from build123d import *

# Parameters (mm, degrees)
ESQUISSE1_W                  = 40
ESQUISSE1_H                  = 10
BOSS_EXTRU_1_DEPTH           = 20
ESQUISSE2_R                  = 1.75
ENL_V_MAT_EXTRU_1_DEPTH      = 1
ENL_V_MAT_EXTRU_1_DEPTH_BACK = 21
ESQUISSE3_R                  = 3.15
ENL_V_MAT_EXTRU_2_DEPTH      = 1
ENL_V_MAT_EXTRU_2_DEPTH_BACK = 11
ESQUISSE4_R                  = 3.65
ENL_V_MAT_EXTRU_3_DEPTH      = 1
CONG_1_R                     = 5


with BuildPart() as part:
    # Esquisse1 → Boss.-Extru.1 (new body)
    with BuildSketch(Plane.XY):
        with Locations((20, 5)):
            Rectangle(ESQUISSE1_W, ESQUISSE1_H)
    extrude(amount=BOSS_EXTRU_1_DEPTH)

    # Esquisse2 → Enlèv. mat.-Extru.1 (cut, two sides)
    with BuildSketch(Plane.XY.offset(20)) as enl_v_mat_extru_1_sk:
        with Locations((20, 5)):
            Circle(ESQUISSE2_R)
        with Locations((11, 5)):
            Circle(ESQUISSE2_R)
        with Locations((29, 5)):
            Circle(ESQUISSE2_R)
    extrude(amount=ENL_V_MAT_EXTRU_1_DEPTH, mode=Mode.SUBTRACT)
    extrude(enl_v_mat_extru_1_sk.sketch, amount=-ENL_V_MAT_EXTRU_1_DEPTH_BACK, mode=Mode.SUBTRACT)

    # Esquisse3 → Enlèv. mat.-Extru.2 (cut, two sides)
    with BuildSketch(Plane(origin=(0, 10, 0), x_dir=(1, 0, 0), z_dir=(0, 1, 0))) as enl_v_mat_extru_2_sk:
        with Locations((5, -10)):
            Circle(ESQUISSE3_R)
        with Locations((35, -10)):
            Circle(ESQUISSE3_R)
    extrude(amount=ENL_V_MAT_EXTRU_2_DEPTH, mode=Mode.SUBTRACT)
    extrude(enl_v_mat_extru_2_sk.sketch, amount=-ENL_V_MAT_EXTRU_2_DEPTH_BACK, mode=Mode.SUBTRACT)

    # Esquisse4 → Enlèv. mat.-Extru.3 (cut)
    with BuildSketch(Plane(origin=(0, 10, 0), x_dir=(1, 0, 0), z_dir=(0, 1, 0))):
        with Locations((5, -10)):
            Circle(ESQUISSE4_R)
        with Locations((35, -10)):
            Circle(ESQUISSE4_R)
    extrude(amount=-ENL_V_MAT_EXTRU_3_DEPTH, mode=Mode.SUBTRACT)

    # Congé1
    cong_1_edges = [part.edges().sort_by_distance(p)[0] for p in [
        (40, 5, 20),
        (0, 5, 20),
        (40, 5, 0),
        (0, 5, 0),
    ]]
    fillet(cong_1_edges, radius=CONG_1_R)


solid = part.part
Work out the finished part from the listing and answer in its coordinate system (mm). A direction names the side the tool comes from. Give positions to 0.01 mm unless a question says otherwise; leave off trailing zeros. Order: outer loops, then holes, each group sorted by start corner. A loop starts at its lowest first (then second) coordinate and runs counter-clockwise, first axis right, second up. Notation, with made-up numbers: (-18, -14.75) -> (10, -14.75) arc R27 ccw to (10, 22.25) -> close; hole circle Ø8 at (-13, 82). An arc over 180 degrees is marked (long way). One line per item, written item: value.
Item 1: Straight lines are drawn through the part: probe 1 along X at (y, z) = (9.5, 10); probe 2 along X at (y, z) = (5.75, 17.5); probe 3 along X at (y, z) = (2.5, 10). For each, find the intervals that lie inside material, in ascending order.
Answer sheet:
probe 1: 0 to 1.35, 8.65 to 31.35, 38.65 to 40
probe 2: 0.67 to 9.42, 12.58 to 18.42, 21.58 to 27.42, 30.58 to 39.33
probe 3: 0 to 1.85, 8.15 to 31.85, 38.15 to 40
Item 2: Find section C-C, the plane x = 11. Give the vertices of the cut face in (y, z), plus the area to 3 significant figures.
Answer sheet:
outline: (0, 0) -> (3.25, 0) -> (3.25, 20) -> (0, 20) -> close; (6.75, 0) -> (10, 0) -> (10, 20) -> (6.75, 20) -> close
area: 130 mm²
Item 3: Find section D-D, the plane y = 7.25. Give the vertices of the cut face in (x, z), plus the area to 3 significant figures.
Answer sheet:
outline: (0, 5) arc R5 ccw to (5, 0) -> (35, 0) arc R5 ccw to (40, 5) -> (40, 15) arc R5 ccw to (35, 20) -> (5, 20) arc R5 ccw to (0, 15) -> close; hole circle Ø6.3 at (5, 10); hole circle Ø6.3 at (35, 10)
area: 716 mm²
Item 4: Find section A-A, the plane z = 10. Give the vertices of the cut face in (x, y), plus the area to 3 significant figures.
Answer sheet:
outline: (0, 0) -> (1.85, 0) -> (1.85, 9) -> (1.35, 9) -> (1.35, 10) -> (0, 10) -> close; (8.15, 0) -> (31.85, 0) -> (31.85, 9) -> (31.35, 9) -> (31.35, 10) -> (8.65, 10) -> (8.65, 9) -> (8.15, 9) -> close; (38.15, 0) -> (40, 0) -> (40, 10) -> (38.65, 10) -> (38.65, 9) -> (38.15, 9) -> close; hole circle Ø3.5 at (11, 5); hole circle Ø3.5 at (20, 5); hole circle Ø3.5 at (29, 5)
area: 243 mm²
Item 5: A flat-ended cylindrical pin translates along its axis: P1, Ø2, axis at x = 33.5, z = 8, coming from the +Y side. Find the tip coordinate at first contact, or state that the pin passes through.
Answer sheet:
P1: y = 9
Item 6: Determine the mould class of faces 3 (the cylindrical face through (11.81, 3.45, 10.14)), 4 (the cylindrical face through (38, 5, 1)), 5 (the cylindrical face through (1, 5, 2)) for opening direction X: released by +X, released by -X, zero draft, split by the parting line, or undercut.
Answer sheet:
face 3: undercut
face 4: released by +X
face 5: released by -X
Item 7: A tool of negligible diameter and unlimited length cuts with its end or side. For faces 1 (the cylindrical face through (6.68, 9.51, 13.24)), 2 (the cylindrical face through (4.59, 4.563, 6.877)), from which of +Z, -Z, +X, -X, +Y, -Y can it reach the whole face along a straight path? Write none if from no direction.
Answer sheet:
face 1: +Y
face 2: +Y, -Y
Item 8: Find section B-B, the plane y = 5. Give the vertices of the cut face in (x, z).
Answer sheet:
outline: (0, 5) arc R5 ccw to (5, 0) -> (9.25, 0) -> (9.25, 20) -> (5, 20) arc R5 ccw to (0, 15) -> close; (12.75, 0) -> (18.25, 0) -> (18.25, 20) -> (12.75, 20) -> close; (21.75, 0) -> (27.25, 0) -> (27.25, 20) -> (21.75, 20) -> close; (30.75, 0) -> (35, 0) arc R5 ccw to (40, 5) -> (40, 15) arc R5 ccw to (35, 20) -> (30.75, 20) -> close; hole circle Ø6.3 at (5, 10); hole circle Ø6.3 at (35, 10)
